Could you check a few things on this model? Use its own coordinates, in mm. A direction names the side the tool comes from. Coordinates: 2 decimals unless noted, no trailing zeros. Write each loop counter-clockwise with the first axis right and the second up, starting at its lowest first coordinate (ties: lowest second). Pieces come first, ordered by that corner, then holes.
Item 1: I want a section at B-B on x = -40. Please give me the cut outline in (y, z), then the cut area to 3 significant figures.
Item 2: I want a section at D-D on z = -58. Please give me the cut outline in (x, y).
Item 3: I want a section at C-C on z = -21. Please give me the cut outline in (x, y) (3 decimals), then the cut area to 3 significant figures.
Item 4: If I drill on probe 1 along Z at (x, y) = (-40.5, 4.75); probe 2 along X at (y, z) = (4, -209.5); probe 3 along X at (y, z) = (5.25, 1), over which ranges is the centre line in solid material (lowest first)?
Item 5: Which directions (+Z, -Z, +X, -X, +Y, -Y) give clear straight access to the entire face, cutting with the end or side of a thin tool? Please do faces 5 (the flat face through (178.402, 4.93, 43.261)), 6 (the flat face through (170.33, 4.93, -36.96)), 7 (the cylindrical face through (-7.4, 4.93, 67.27)).
Item 6: I want a section at A-A on z = -204. Please give me the cut outline in (x, y), then the cut area to 3 significant figures.
Item 7: Thinking about a two-plate mould opening in Z: for faces 1 (the flat face through (59, 10, -44)), 2 (the flat face through (-65.506, 4.93, 43.382)), 3 (the flat face through (7, 5, 84.952)), 4 (the flat face through (106.035, 4.93, -168.138)), which applies, +Z half, -Z half, draft (parallel to the pull), parting line (faces both ways), or undercut?
Item 8: For P1, Ø3, axis at y = 6, z = 36.5, coming from the +X side; P2, Ø1, axis at x = 20.5, z = -192.5, coming from the -Y side; P3, Ø3, axis at y = 4, z = 34, coming from the -X side; P4, Ø5, axis at x = 48.5, y = 3, coming from the -Z side, each with a flat end and sliding along its axis, tell me the tip position at first contact or that it passes through.
from build123d import *

# Parameters (mm, degrees)
BOSS_EXTRU_1_DEPTH = 10


with BuildPart() as part:
    # Esquisse2 → Boss.-Extru.1 (new body)
    with BuildSketch(Plane(origin=(0, 0, 0), x_dir=(1, 0, 0), z_dir=(0, 1, 0))):
        with BuildLine():
            Line((36.413113552, 132.966619465), (76.413113552, 132.966619465))
            Line((76.413113552, 132.966619465), (75.069459937, 210.531035708))
            Line((75.069459937, 210.531035708), (85.069084249, 210.617716914))
            Line((85.069084249, 210.617716914), (84.813374692, 240.116608632))
            Line((84.813374692, 240.116608632), (102.812698453, 240.272634802))
            ThreePointArc((102.812698453, 240.272634802), (89.604268477, 211.329810699), (102.868184053, 182.412372481))
            Line((102.868184053, 182.412372481), (91.624672702, 167.096255072))
            Line((91.624672702, 167.096255072), (100.49189857, 160.586853763))
            Line((100.49189857, 160.586853763), (111.735409922, 175.902971172))
            ThreePointArc((111.735409922, 175.902971172), (129.846153012, 172.469977356), (147.507194899, 177.749377064))
            Line((147.507194899, 177.749377064), (158.112115685, 159.623824517))
            ThreePointArc((158.112115685, 159.623824517), (141.072313982, 138.74483792), (141.863284971, 111.806736869))
            Line((141.863284971, 111.806736869), (125.463975524, 102.211808539))
            Line((125.463975524, 102.211808539), (131.01893403, 92.717471491))
            Line((131.01893403, 92.717471491), (147.418243478, 102.312399821))
            ThreePointArc((147.418243478, 102.312399821), (170.51388989, 88.424345956), (197.063848919, 93.048910681))
            Line((197.063848919, 93.048910681), (207.668769705, 74.923358135))
            ThreePointArc((207.668769705, 74.923358135), (194.413310744, 62.114093146), (188.532513668, 44.644099226))
            Line((188.532513668, 44.644099226), (169.671901636, 42.346858754))
            Line((169.671901636, 42.346858754), (171.001882962, 31.427557051))
            Line((171.001882962, 31.427557051), (189.862494994, 33.724797523))
            ThreePointArc((189.862494994, 33.724797523), (208.572406926, 7.993709614), (240.274776322, 5.32735176))
            Line((240.274776322, 5.32735176), (231.319855268, -10.287045088))
            Line((231.319855268, -10.287045088), (205.729593768, 4.389075528))
            Line((205.729593768, 4.389075528), (200.754637626, -4.285589387))
            Line((200.754637626, -4.285589387), (133.168524557, 34.475325478))
            Line((133.168524557, 34.475325478), (113.268699993, -0.223334184))
            Line((113.268699993, -0.223334184), (180.854813062, -38.984249048))
            Line((180.854813062, -38.984249048), (175.879856921, -47.658913964))
            Line((175.879856921, -47.658913964), (201.470118422, -62.33503458))
            Line((201.470118422, -62.33503458), (192.515197368, -77.949431428))
            ThreePointArc((192.515197368, -77.949431428), (174.204229484, -51.93293388), (142.546738059, -48.778108028))
            Line((142.546738059, -48.778108028), (135.004997884, -31.339009567))
            Line((135.004997884, -31.339009567), (124.908677722, -35.705280195))
            Line((124.908677722, -35.705280195), (132.450417897, -53.144378656))
            ThreePointArc((132.450417897, -53.144378656), (120.34147001, -67.042502374), (115.979474134, -84.952205157))
            Line((115.979474134, -84.952205157), (94.979474134, -84.952205157))
            ThreePointArc((94.979474134, -84.952205157), (85.563406447, -59.700975629), (61.913113552, -46.780040317))
            Line((61.913113552, -46.780040317), (61.913113552, -27.780040317))
            Line((61.913113552, -27.780040317), (50.913113552, -27.780040317))
            Line((50.913113552, -27.780040317), (50.913113552, -46.780040317))
            ThreePointArc((50.913113552, -46.780040317), (27.262820657, -59.700975629), (17.84675297, -84.952205157))
            Line((17.84675297, -84.952205157), (-3.15324703, -84.952205157))
            ThreePointArc((-3.15324703, -84.952205157), (-7.515242906, -67.042502374), (-19.624190793, -53.144378656))
            Line((-19.624190793, -53.144378656), (-12.082450618, -35.705280195))
            Line((-12.082450618, -35.705280195), (-22.17877078, -31.339009567))
            Line((-22.17877078, -31.339009567), (-29.720510955, -48.778108028))
            ThreePointArc((-29.720510955, -48.778108028), (-61.37800238, -51.93293388), (-79.688970264, -77.949431428))
            Line((-79.688970264, -77.949431428), (-88.643891318, -62.33503458))
            Line((-88.643891318, -62.33503458), (-63.053629817, -47.658913964))
            Line((-63.053629817, -47.658913964), (-68.028585958, -38.984249048))
            Line((-68.028585958, -38.984249048), (-0.442472889, -0.223334184))
            Line((-0.442472889, -0.223334184), (-20.342297454, 34.475325478))
            Line((-20.342297454, 34.475325478), (-87.928410523, -4.285589387))
            Line((-87.928410523, -4.285589387), (-92.903366664, 4.389075528))
            Line((-92.903366664, 4.389075528), (-118.493628164, -10.287045088))
            Line((-118.493628164, -10.287045088), (-127.448549218, 5.32735176))
            ThreePointArc((-127.448549218, 5.32735176), (-95.746179823, 7.993709614), (-77.03626789, 33.724797523))
            Line((-77.03626789, 33.724797523), (-58.175655858, 31.427557051))
            Line((-58.175655858, 31.427557051), (-56.845674532, 42.346858754))
            Line((-56.845674532, 42.346858754), (-75.706286564, 44.644099226))
            ThreePointArc((-75.706286564, 44.644099226), (-81.58708364, 62.114093146), (-94.842542601, 74.923358135))
            Line((-94.842542601, 74.923358135), (-84.237621815, 93.048910681))
            ThreePointArc((-84.237621815, 93.048910681), (-57.687662786, 88.424345956), (-34.592016374, 102.312399821))
            Line((-34.592016374, 102.312399821), (-18.192706927, 92.717471491))
            Line((-18.192706927, 92.717471491), (-12.63774842, 102.211808539))
            Line((-12.63774842, 102.211808539), (-29.037057867, 111.806736869))
            ThreePointArc((-29.037057867, 111.806736869), (-28.246086878, 138.74483792), (-45.285888581, 159.623824517))
            Line((-45.285888581, 159.623824517), (-34.680967795, 177.749377064))
            ThreePointArc((-34.680967795, 177.749377064), (-17.019925908, 172.469977356), (1.090817182, 175.902971172))
            Line((1.090817182, 175.902971172), (12.334328534, 160.586853763))
            Line((12.334328534, 160.586853763), (21.201554402, 167.096255072))
            Line((21.201554402, 167.096255072), (9.95804305, 182.412372481))
            ThreePointArc((9.95804305, 182.412372481), (23.221958626, 211.329810699), (10.013528651, 240.272634802))
            Line((10.013528651, 240.272634802), (28.012852411, 240.116608632))
            Line((28.012852411, 240.116608632), (27.757142855, 210.617716914))
            Line((27.757142855, 210.617716914), (37.756767167, 210.531035708))
            Line((37.756767167, 210.531035708), (36.413113552, 132.966619465))
        make_face()
    extrude(amount=BOSS_EXTRU_1_DEPTH)


solid = part.part
Response values:
1. outline: (0, -168.66) - (10, -168.66) - (10, -155.9) - (0, -155.9) - close; (0, -96.77) - (10, -96.77) - (10, -23.2) - (0, -23.2) - close; (0, 22.91) - (10, 22.91) - (10, 46.78) - (0, 46.78) - close
1. area: 1,100 mm2
2. outline: (-79.32, 0) - (192.15, 0) - (192.15, 10) - (-79.32, 10) - close
3. outline: (-82.115, 0) - (-43.839, 0) - (-43.839, 10) - (-82.115, 10) - close; (-12.614, 0) - (125.44, 0) - (125.44, 10) - (-12.614, 10) - close; (156.665, 0) - (194.941, 0) - (194.941, 10) - (156.665, 10) - close
3. area: 2,150 mm2
4. probe 1: z = -167.8 to -156.32, -96.36 to -22.91, 23.2 to 46.75
4. probe 2: x = 23.18 to 37.74, 75.09 to 89.65
4. probe 3: x = -123.82 to -102.3, -89.81 to -82.2, -1.8 to 114.62, 195.03 to 202.64, 215.13 to 236.65
5. face 5: +X, +Y, -Y
5. face 6: +Y, -Y
5. face 7: +Z, +Y, -Y
6. outline: (22.51, 0) - (37.64, 0) - (37.64, 10) - (22.51, 10) - close; (75.18, 0) - (90.32, 0) - (90.32, 10) - (75.18, 10) - close
6. area: 303 mm2
7. face 1: draft
7. face 2: undercut
7. face 3: +Z half
7. face 4: undercut
8. P1: stops at x = 179.14
8. P2: stops at y = 0
8. P3: stops at x = -61.95
8. P4: stops at z = -132.97
